Read the model definition and answer for the solid it produces. Units are mm, in the model's axes. A direction names the side the tool comes from. Coordinates: 2 decimals unless noted, no trailing zeros. Order: outer loops, then holes, each group sorted by start corner. A loop starts at its lowest first (then second) coordinate and runs counter-clockwise, first axis right, second up.
Autodesk Inventor part; units mm, degrees
ref_plane "YZ Plane" through (0, 0, 0) normal (1, 0, 0) x (0, 1, 0)
ref_plane "XZ Plane" through (0, 0, 0) normal (0, 1, 0) x (-1, 0, 0)
ref_plane "XY Plane" through (0, 0, 0) normal (0, 0, 1) x (1, 0, 0)
sketch "スケッチ1" plane through (0, 0, 0) normal (0, 1, 0) x (-1, 0, 0)
  circle A0 centre (0, 0) radius 2.75
  dimension "d0" = 5.5
extrude "押し出し1" add sketch "スケッチ1" along normal blind 3
sketch "スケッチ2" plane through (0, 0, 0) normal (0, -1, 0) x (1, 0, 0)
  circle A0 centre (0, 0) radius 1.5
  dimension "d3" = 3
extrude "押し出し2" add sketch "スケッチ2" along normal blind 12
fillet "フィレット1" radius 0.5 1 edges at (2.75, 3, 0)
fillet "フィレット1" radius 0.2 1 edges at (2.75, 0, 0)
sketch "スケッチ3" plane through (0, 3, 0) normal (0, 1, 0) x (1, 0, 0)
  line L0 (0, 1.4434) -> (-1.25, 0.7217)
  line L1 (-1.25, 0.7217) -> (-1.25, -0.7217)
  line L2 (-1.25, -0.7217) -> (0, -1.4434)
  line L3 (0, -1.4434) -> (1.25, -0.7217)
  line L4 (1.25, -0.7217) -> (1.25, 0.7217)
  line L5 (1.25, 0.7217) -> (0, 1.4434)
  line L6 (0, 1.4434) -> (0, -1.4434) construction
  circle A0 centre (0, 0) radius 1.4434 construction
  dimension "d12" = 2.5
extrude "押し出し3" cut sketch "スケッチ3" against normal blind 2
thread "ねじ1"
properties part number "M3-CapScrew"
Q1. Each of these flat-tipped pins is pushed along its axis until it touches: P1, Ø1.2, axis at y = 2.5, z = 0.5, coming from the -X side; P2, Ø3, axis at x = 1.5, y = -9.5, coming from the -Z side. Where does it stop, or does it pass through?
Q2. The part is cut by section A-A, the plane z = 0. Determine the outline of the cut face in (x, y).
Q3. Determine the mould class of faces 1 (the cylindrical face through (0.596, 1.334, 2.685)), 2 (the flat face through (-2, 0, 0)), 3 (the flat face through (-1.25, 2, 0)) for opening direction X: +X half, -X half, draft (parallel to the pull), parting line (faces both ways), or undercut.
Q4. The part is cut by section B-B, the plane y = -7.25. Determine the outline of the cut face in (x, z).
Q5. Straight lines are drawn through the part: L1, parallel to Z at x = -1, y = 1.5; L2, parallel to Z at x = 0.4, y = -7; L3, parallel to Y at x = 0.5, z = 2.2. For each, find the intervals that lie inside material, in ascending order.
Q6. Which of the six approach directions +Z, -Z, +X, -X, +Y, -Y give full straight-line access (tool end or side, diameter ignored) to faces 4 (the cylindrical face through (-1.5, -5.92, -0.07)), 5 (the flat face through (-0.63, 2.01, 1.08)), 6 (the flat face through (-1.5, 3, 0))?
Q7. The part is cut by section C-C, the plane y = 0.5. Determine the outline of the cut face in (x, z).
Computed values:
1. P1: stops at x = -2.75
1. P2: stops at z = -1.5
2. outline: (-2.75, 0.2) arc R0.2 ccw to (-2.55, 0) - (-1.5, 0) - (-1.5, -12) - (1.5, -12) - (1.5, 0) - (2.55, 0) arc R0.2 ccw to (2.75, 0.2) - (2.75, 2.5) arc R0.5 ccw to (2.25, 3) - (1.25, 3) - (1.25, 1) - (-1.25, 1) - (-1.25, 3) - (-2.25, 3) arc R0.5 ccw to (-2.75, 2.5) - close
3. face 1: parting line
3. face 2: draft
3. face 3: undercut
4. outline: circle Ø3 at (0, 0)
5. L1: z = -2.56 to -0.87, 0.87 to 2.56
5. L2: z = -1.45 to 1.45
5. L3: y = 0 to 3
6. face 4: -Y
6. face 5: +Y
6. face 6: +Z, -Z, +X, -X, +Y
7. outline: circle Ø5.5 at (0, 0)
